from build123d import *

# Parameters (mm, degrees)
F0_R     = 25.4
F0_R_2   = 3.125
F1_DEPTH = 5
F2_R     = 6.031593
F3_DEPTH = 8
F4_R     = 3
F5_DEPTH = 8.001


with BuildPart() as f1:
    # F0 (on Top) → F1 (new body)
    with BuildSketch(Plane.XY):
        Circle(F0_R)
        with BuildLine():
            ThreePointArc((-10.88453, -17.158945), (-11.801786, -15.683608), (-11.218679, -14.04716))
            Line((-11.218679, -14.04716), (-6.139343, -9.030124))
            ThreePointArc((-6.139343, -9.030124), (-5.086026, -8.484282), (-3.908805, -8.631157))
            ThreePointArc((-3.908805, -8.631157), (-3.625926, -8.753759), (-3.339207, -8.867092))
            ThreePointArc((-3.339207, -8.867092), (-2.40293, -9.595657), (-2.044091, -10.726433))
            Line((-2.044091, -10.726433), (-2.000038, -17.865646))
            ThreePointArc((-2.000038, -17.865646), (-2.744862, -19.435109), (-4.436681, -19.829732))
            ThreePointArc((-4.436681, -19.829732), (-7.776127, -18.773232), (-10.88453, -17.158945))
        make_face(mode=Mode.SUBTRACT)
        with BuildLine():
            ThreePointArc((-19.829732, -4.436681), (-19.435109, -2.744862), (-17.865646, -2.000038))
            Line((-17.865646, -2.000038), (-10.726433, -2.044091))
            ThreePointArc((-10.726433, -2.044091), (-9.595657, -2.40293), (-8.867092, -3.339207))
            ThreePointArc((-8.867092, -3.339207), (-8.753759, -3.625926), (-8.631157, -3.908805))
            ThreePointArc((-8.631157, -3.908805), (-8.484282, -5.086026), (-9.030124, -6.139343))
            Line((-9.030124, -6.139343), (-14.04716, -11.218679))
            ThreePointArc((-14.04716, -11.218679), (-15.683608, -11.801786), (-17.158945, -10.88453))
            ThreePointArc((-17.158945, -10.88453), (-18.773232, -7.776127), (-19.829732, -4.436681))
        make_face(mode=Mode.SUBTRACT)
        Circle(F0_R_2, mode=Mode.SUBTRACT)
        with BuildLine():
            ThreePointArc((4.436681, -19.829732), (2.744862, -19.435109), (2.000038, -17.865646))
            Line((2.000038, -17.865646), (2.044091, -10.726433))
            ThreePointArc((2.044091, -10.726433), (2.40293, -9.595657), (3.339207, -8.867092))
            ThreePointArc((3.339207, -8.867092), (3.625926, -8.753759), (3.908805, -8.631157))
            ThreePointArc((3.908805, -8.631157), (5.086026, -8.484282), (6.139343, -9.030124))
            Line((6.139343, -9.030124), (11.218679, -14.04716))
            ThreePointArc((11.218679, -14.04716), (11.801786, -15.683608), (10.88453, -17.158945))
            ThreePointArc((10.88453, -17.158945), (7.776127, -18.773232), (4.436681, -19.829732))
        make_face(mode=Mode.SUBTRACT)
        with BuildLine():
            ThreePointArc((17.158945, -10.88453), (15.683608, -11.801786), (14.04716, -11.218679))
            Line((14.04716, -11.218679), (9.030124, -6.139343))
            ThreePointArc((9.030124, -6.139343), (8.484282, -5.086026), (8.631157, -3.908805))
            ThreePointArc((8.631157, -3.908805), (8.753759, -3.625926), (8.867092, -3.339207))
            ThreePointArc((8.867092, -3.339207), (9.595657, -2.40293), (10.726433, -2.044091))
            Line((10.726433, -2.044091), (17.865646, -2.000038))
            ThreePointArc((17.865646, -2.000038), (19.435109, -2.744862), (19.829732, -4.436681))
            ThreePointArc((19.829732, -4.436681), (18.773232, -7.776127), (17.158945, -10.88453))
        make_face(mode=Mode.SUBTRACT)
        with BuildLine():
            ThreePointArc((-17.158945, 10.88453), (-15.683608, 11.801786), (-14.04716, 11.218679))
            Line((-14.04716, 11.218679), (-9.030124, 6.139343))
            ThreePointArc((-9.030124, 6.139343), (-8.484282, 5.086026), (-8.631157, 3.908805))
            ThreePointArc((-8.631157, 3.908805), (-8.753759, 3.625926), (-8.867092, 3.339207))
            ThreePointArc((-8.867092, 3.339207), (-9.595657, 2.40293), (-10.726433, 2.044091))
            Line((-10.726433, 2.044091), (-17.865646, 2.000038))
            ThreePointArc((-17.865646, 2.000038), (-19.435109, 2.744862), (-19.829732, 4.436681))
            ThreePointArc((-19.829732, 4.436681), (-18.773232, 7.776127), (-17.158945, 10.88453))
        make_face(mode=Mode.SUBTRACT)
        with BuildLine():
            ThreePointArc((-10.88453, 17.158945), (-7.776127, 18.773232), (-4.436681, 19.829732))
            ThreePointArc((-4.436681, 19.829732), (-2.744862, 19.435109), (-2.000038, 17.865646))
            Line((-2.000038, 17.865646), (-2.044091, 10.726433))
            ThreePointArc((-2.044091, 10.726433), (-2.40293, 9.595657), (-3.339207, 8.867092))
            ThreePointArc((-3.339207, 8.867092), (-3.625926, 8.753759), (-3.908805, 8.631157))
            ThreePointArc((-3.908805, 8.631157), (-5.086026, 8.484282), (-6.139343, 9.030124))
            Line((-6.139343, 9.030124), (-11.218679, 14.04716))
            ThreePointArc((-11.218679, 14.04716), (-11.801786, 15.683608), (-10.88453, 17.158945))
        make_face(mode=Mode.SUBTRACT)
        with BuildLine():
            ThreePointArc((19.829732, 4.436681), (19.435109, 2.744862), (17.865646, 2.000038))
            Line((17.865646, 2.000038), (10.726433, 2.044091))
            ThreePointArc((10.726433, 2.044091), (9.595657, 2.40293), (8.867092, 3.339207))
            ThreePointArc((8.867092, 3.339207), (8.753759, 3.625926), (8.631157, 3.908805))
            ThreePointArc((8.631157, 3.908805), (8.484282, 5.086026), (9.030124, 6.139343))
            Line((9.030124, 6.139343), (14.04716, 11.218679))
            ThreePointArc((14.04716, 11.218679), (15.683608, 11.801786), (17.158945, 10.88453))
            ThreePointArc((17.158945, 10.88453), (18.773232, 7.776127), (19.829732, 4.436681))
        make_face(mode=Mode.SUBTRACT)
        with BuildLine():
            Line((2.044091, 10.726433), (2.000038, 17.865646))
            ThreePointArc((2.000038, 17.865646), (2.744862, 19.435109), (4.436681, 19.829732))
            ThreePointArc((4.436681, 19.829732), (7.776127, 18.773232), (10.88453, 17.158945))
            ThreePointArc((10.88453, 17.158945), (11.801786, 15.683608), (11.218679, 14.04716))
            Line((11.218679, 14.04716), (6.139343, 9.030124))
            ThreePointArc((6.139343, 9.030124), (5.086026, 8.484282), (3.908805, 8.631157))
            ThreePointArc((3.908805, 8.631157), (3.625926, 8.753759), (3.339207, 8.867092))
            ThreePointArc((3.339207, 8.867092), (2.40293, 9.595657), (2.044091, 10.726433))
        make_face(mode=Mode.SUBTRACT)
    extrude(amount=F1_DEPTH)

    # F2 (on Top) → F3 (join)
    with BuildSketch(Plane.XY):
        Circle(F2_R)
    extrude(amount=F3_DEPTH)

    # F4 (on face) → F5 (cut, through all)
    with BuildSketch(Plane.XY.offset(8)):
        Circle(F4_R)
    extrude(amount=-F5_DEPTH, mode=Mode.SUBTRACT)

    # F6 (on Right) → F7 (revolve, cut)
    with BuildSketch(Plane.YZ):
        Polygon((25.457971, 0.902619), (25.4, 2.402619), (23.4, 2.402619), align=None)
        Polygon((23.4, 2.402619), (25.4, 2.402619), (25.457971, 3.902619), align=None)
    revolve(axis=Axis((0, 0, 8.098846), (0, 0, -1)), mode=Mode.SUBTRACT)


solid = f1.part
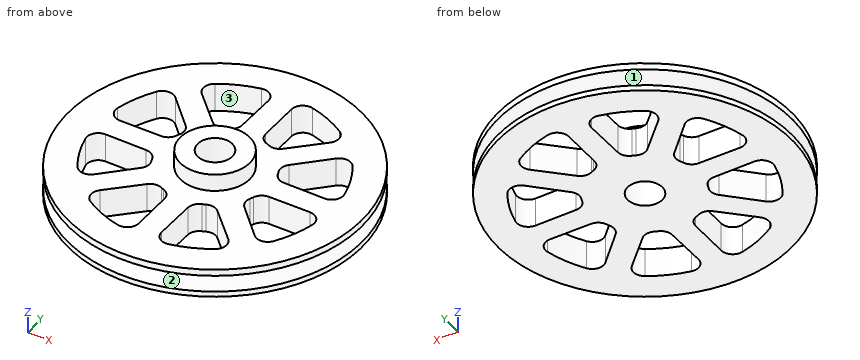
Can you work these out from the model? Positions are in its coordinate system, mm. Face numbers are marked on the shaded views. Coordinates: 2 decimals unless noted, no trailing zeros. Order: outer loops, then holes, each group sorted by start corner. A loop starts at its lowest first (then second) coordinate and runs counter-clockwise, first axis right, second up. Notation, with made-up numbers: (3, -15.75) - (60, -15.75) arc R23 ccw to (60, 11.25) - close; hole circle Ø5 at (-7, -27.75). An arc over 180 degrees is marked (long way). Answer as a JSON object with one key per item and string values. Group by question number.
Q1. I need wall thicknesses on line 1 (Y direction, x = 0, z = 5.25); line 2 (Y direction, x = -5.5, z = 4.25); line 3 (X direction, y = -8, z = 1.25). Which ranges of each line are inside material? Lowest first, please. Write a range as from..to.
Q2. Imagine slicing it at A-A (y = 0). Please give me the cut outline in (x, z), and give its area (3 significant figures).
Q3. Imagine slicing it at C-C (y = -19). Give the number of separate pieces and of enclosed holes in the cut face, and give its area (3 significant figures).
Q4. Imagine slicing it at B-B (z = 6.75). Please give me the cut outline in (x, y), and give its area (3 significant figures).
Q5. We'd pull the mould along Z, two halves only. Please class the marked faces 1, 2 and 3: +Z half, -Z half, draft (parallel to the pull), parting line (faces both ways), or undercut.
Q6. Will these pins go through, and if not, where does the flat tip stop? P1, Ø5, axis at x = 0, y = 0, coming from the -Z side; P2, Ø4, axis at y = -5, z = 6.5, coming from the +X side; P3, Ø3, axis at y = -14.5, z = 3, coming from the -X side; P4, Ø2, axis at x = 18.5, z = 2.5, coming from the +Y side.
Determined:
{
 "1": {"line 1": "y = -6.03..-3, 3..6.03", "line 2": "y = -24.8..-19.56, -8.61..8.61, 19.56..24.8", "line 3": "x = -23.67..-18.68, -10.87..10.87, 18.68..23.67"},
 "2": {"outline": "(-25.4, 0) - (-3, 0) - (-3, 8) - (-6.03, 8) - (-6.03, 5) - (-25.4, 5) - (-25.4, 3.86) - (-23.4, 2.4) - (-25.4, 0.94) - close; (3, 0) - (25.4, 0) - (25.4, 0.94) - (23.4, 2.4) - (25.4, 3.86) - (25.4, 5) - (6.03, 5) - (6.03, 8) - (3, 8) - close", "area": "236 mm2"},
 "3": {"separate pieces": "3", "enclosed holes": "0", "area": "111 mm2"},
 "4": {"outline": "circle Ø12.06 at (0, 0); hole circle Ø6 at (0, 0)", "area": "86.0 mm2"},
 "5": {"face 1": "undercut", "face 2": "undercut", "face 3": "draft"},
 "6": {"P1": "passes through", "P2": "stops at x = 25.13", "P3": "stops at x = -21.66", "P4": "stops at y = 16.95"}
}
